Model file for the job. Use its own axes, mm. A direction names the side the tool comes from. Give positions to 0.01 mm unless a question says otherwise; leave off trailing zeros. Order: outer loops, then holes, each group sorted by start corner. A loop starts at its lowest first (then second) coordinate and runs counter-clockwise, first axis right, second up. Notation, with made-up numbers: M 77.5,-31 L 97.5,-31 A12 cw 97.5,-12 Z; hole C 24,16.5 d5. An arc over 180 degrees is marked long. Return JSON: item names as keys, results as strings. Group by question number.
1. Two-plate mould, pull along Y, no slides. Class faces 1 (the face through (1, 3, 0)), 2 (the face through (0, 0, 4)), 3 (the face through (-3.746, -0.165, 1.202)): released by +Y, released by -Y, zero draft, split by the parting line, or undercut.
2. Pin check, flat tips, straight feed: pin 1 (4 mm diameter, centred on x = 1, y = -1.5, fed in from +Z); pin 2 (2 mm diameter, centred on x = -2.5, z = 8, fed in from -Y); pin 3 (2.5 mm diameter, centred on x = 0, y = 0, fed in from +Z); pin 4 (1 mm diameter, centred on y = -1, z = 2, fed in from -X). Stop position of each tip, or through.
3. Slice it at B-B on z = 0.75. List the corners of the cut face in (x, y), then the cut area to 3 significant figures.
4. Wall check: probe 1 along Y at (x, z) = (0, 1.7); probe 2 along Y at (x, z) = (-2, 2.75); probe 3 along X at (y, z) = (0.25, 5.75). Give the ranges that are in metal, low to high. Write a range as [from, to].
5. Slice it at A-A on z = 7.5. List the corners of the cut face in (x, y) (3 decimals), then the cut area to 3 significant figures.
6. 3-axis set-ups, long thin cutter, end or side, ignore diameter. For faces 4 (the face through (-1.13, 0.87, 6.07)), 5 (the face through (-0.29, -2.23, 1.66)): which of +Z, -Z, +X, -X, +Y, -Y reach the whole face in a straight line?
Autodesk Inventor part; units mm, degrees
ref_plane "YZ Plane" through (0, 0, 0) normal (1, 0, 0) x (0, 1, 0)
ref_plane "XZ Plane" through (0, 0, 0) normal (0, 1, 0) x (-1, 0, 0)
ref_plane "XY Plane" through (0, 0, 0) normal (0, 0, 1) x (1, 0, 0)
sketch "Szkic1" plane through (0, 0, 0) normal (0, 0, 1) x (1, 0, 0)
  circle A0 centre (0, 0) radius 2.25
  circle A1 centre (0, 0) radius 3.75
  dimension "d0" = 4.5
  dimension "d1" = 1.5
extrude "Wyciągnięcie proste1" add sketch "Szkic1" along normal blind 3
sketch "Szkic2" plane through (0, 0, 3) normal (0, 0, 1) x (1, 0, 0)
  circle A0 centre (0, 0) radius 3.75
  circle A1 centre (0, 0) radius 2.25
extrude "Wyciągnięcie proste2" add sketch "Szkic2" along normal blind 1 contours A0 | A1
sketch "Szkic3" plane through (0, 0, 4) normal (0, 0, 1) x (1, 0, 0)
  circle A0 centre (0, 0) radius 1.425
  circle A1 centre (0, 0) radius 3
  dimension "d6" = 2.85
  dimension "d7" = 6
extrude "Wyciągnięcie proste3" add sketch "Szkic3" along normal blind 5
fillet "Zaokrąglenie1" radius 2 2 edges at (-3.75, 0, 4) (-3, 0, 4)
chamfer "Faza1" distance 0.8 angle 45 1 edges at (-1.425, 0, 9)
chamfer "Faza2" distance 0.35 angle 45 1 edges at (-2.25, 0, 0)
properties part number "MagnetHolder"
Result:
{
 "1": {"face 1": "zero draft", "face 2": "undercut", "face 3": "split by the parting line"},
 "2": {"pin 1": "stops at z = 9", "pin 2": "stops at y = -2.6", "pin 3": "stops at z = 4", "pin 4": "stops at x = -3.72"},
 "3": {"outline": "C 0,0 d7.5; hole C 0,0 d4.5", "area": "28.3 mm2"},
 "4": {"probe 1": "y = [-3.75, -2.25], [2.25, 3.75]", "probe 2": "y = [-3.14, -1.03], [1.03, 3.14]", "probe 3": "x = [-2.99, -1.4], [1.4, 2.99]"},
 "5": {"outline": "C 0,0 d6; hole C 0,0 d2.85", "area": "21.9 mm2"},
 "6": {"face 4": "+Z", "face 5": "-Z"}
}
